from build123d import *

# Parameters (mm, degrees)
SKETCH1_W                                            = 69.24
SKETCH1_H                                            = 132.04
BOSS_EXTRUDE1_DEPTH                                  = 1.2192
CSK_FOR_M3_CROSS_COUNTERSUNK_HEAD_SCREW1_D           = 3.4
CSK_FOR_M3_CROSS_COUNTERSUNK_HEAD_SCREW1_DEPTH       = 70.76
CSK_FOR_M3_CROSS_COUNTERSUNK_HEAD_SCREW1_CSINK_D     = 6
CSK_FOR_M3_CROSS_COUNTERSUNK_HEAD_SCREW1_CSINK_ANGLE = 92
CSK_FOR_M3_CROSS_COUNTERSUNK_HEAD_SCREW1_TIP         = 1.021463052


with BuildPart() as part:
    # Sketch1 → Boss-Extrude1 (new body)
    with BuildSketch(Plane(origin=(0, 0, 0), x_dir=(1, 0, 0), z_dir=(0, 1, 0))):
        with Locations((34.62, 66.02)):
            Rectangle(SKETCH1_W, SKETCH1_H)
    extrude(amount=BOSS_EXTRUDE1_DEPTH)

    # CSK for M3 Cross Countersunk Head Screw1
    with Locations(Plane(origin=(0, 1.2192, 0), x_dir=(1, 0, 0), z_dir=(0, 1, 0))):
        with Locations((65.74, 112.04), (65.74, 20)):
            CounterSinkHole(CSK_FOR_M3_CROSS_COUNTERSUNK_HEAD_SCREW1_D / 2, CSK_FOR_M3_CROSS_COUNTERSUNK_HEAD_SCREW1_CSINK_D / 2, depth=CSK_FOR_M3_CROSS_COUNTERSUNK_HEAD_SCREW1_DEPTH, counter_sink_angle=CSK_FOR_M3_CROSS_COUNTERSUNK_HEAD_SCREW1_CSINK_ANGLE)
            with Locations((0, 0, -(CSK_FOR_M3_CROSS_COUNTERSUNK_HEAD_SCREW1_DEPTH + CSK_FOR_M3_CROSS_COUNTERSUNK_HEAD_SCREW1_TIP / 2))):  # 118° drill point
                Cone(0, CSK_FOR_M3_CROSS_COUNTERSUNK_HEAD_SCREW1_D / 2, CSK_FOR_M3_CROSS_COUNTERSUNK_HEAD_SCREW1_TIP, mode=Mode.SUBTRACT)


solid = part.part
Design review of the part built by this model. Coordinates are the model's own, in mm. Round coordinates to 2 decimals unless told otherwise and drop trailing zeros. Write each loop counter-clockwise with the first axis right and the second up, starting at its lowest first coordinate (ties: lowest second). Pieces come first, ordered by that corner, then holes. Notation, with made-up numbers: (-13, -32) - (36, -32) arc R5 ccw to (36, -26) - close; hole circle Ø4 at (-4.75, 55.25). An arc over 180 degrees is marked (long way). Return JSON: item names as keys, results as strings. Group by question number.
Item 1: We need section A-A on x = 65.74. Write out the cut boundary in (y, z), and give its area (3 significant figures).
Item 2: Insertion check: P1, Ø10, axis at x = 32, z = -81.5, coming from the -Y side. The pin has a flat end and moves straight along its axis. Give the tip position at first contact, or say it passes through.
Item 3: For probe 1 along Z at (x, y) = (66.5, 0.35); probe 2 along X at (y, z) = (1, -18), list the stretches that pass through material, from the lowest coordinate up. Write a range as [from, to].
Item 4: We need section B-B on z = -20. Write out the cut boundary in (x, y), and give its area (3 significant figures).
Model answer:
{
 "1": {"outline": "(0, -132.04) - (1.22, -132.04) - (1.22, -115.04) - (0, -113.78) - close; (0, -110.3) - (1.22, -109.04) - (1.22, -23) - (0, -21.74) - close; (0, -18.26) - (1.22, -17) - (1.22, 0) - (0, 0) - close", "area": "149 mm²"},
 "2": {"P1": "stops at y = 0"},
 "3": {"probe 1": "z = [-132.04, -114], [-110.08, -21.96], [-18.04, 0]", "probe 2": "x = [0, 63.82], [67.66, 69.24]"},
 "4": {"outline": "(0, 0) - (64, 0) - (62.74, 1.22) - (0, 1.22) - close; (67.48, 0) - (69.24, 0) - (69.24, 1.22) - (68.74, 1.22) - close", "area": "78.6 mm²"}
}
